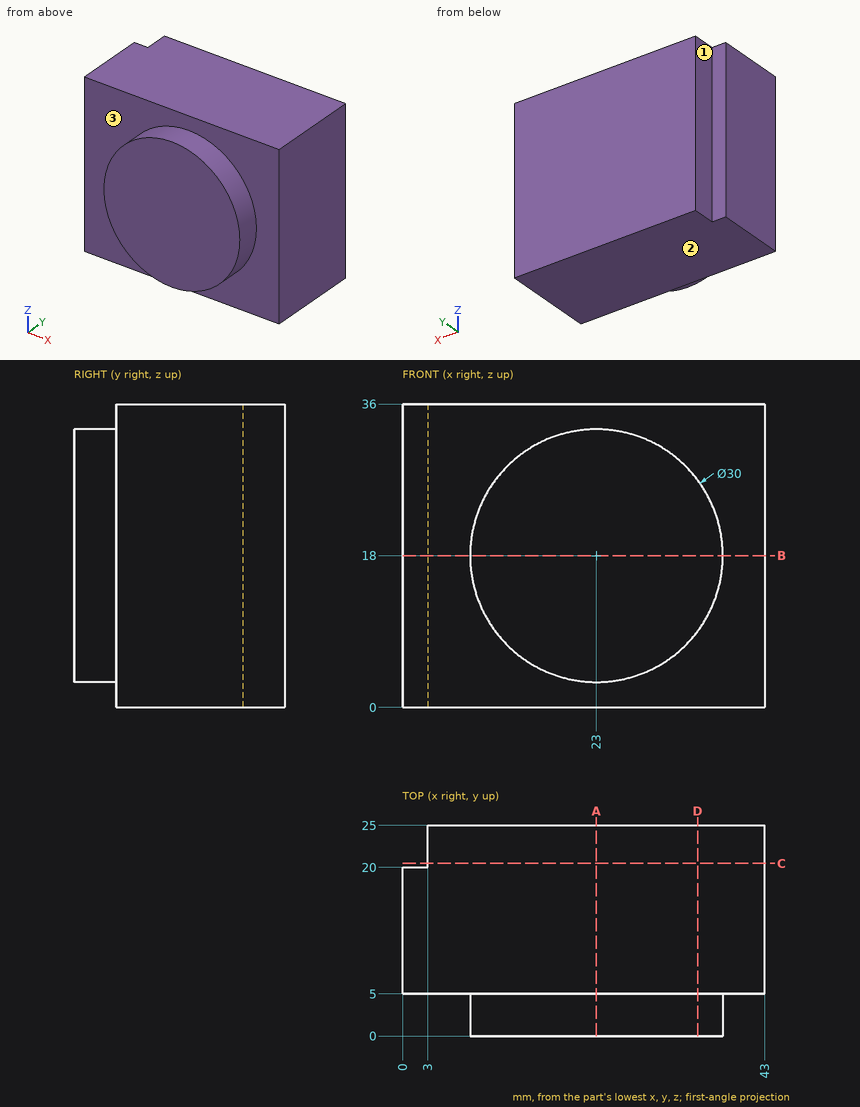
Can you work these out from the drawing? Everything is in mm from the part's minimum corner. A direction names the side the tool comes from. Coordinates: 2 decimals unless noted, no trailing zeros. Loops run counter-clockwise (first coordinate to the right, second up) from the corner with the lowest first, then second, coordinate; pieces in that order, holes last. Notation, with made-up numbers: (-22.75, 17.25) -> (-6.75, 17.25) arc R16 ccw to (-6.75, 40.25) -> close; hole circle Ø9 at (33.25, 71). An arc over 180 degrees is marked (long way). Return JSON: item names as keys, results as strings.
1) If we section it at B-B, the plane z = 18: Write out the boundary of the cut face in (x, y), then the cut area to 3 significant figures.
Results below:
{"outline": "(0, 5) -> (8, 5) -> (8, 0) -> (38, 0) -> (38, 5) -> (43, 5) -> (43, 25) -> (3, 25) -> (3, 20) -> (0, 20) -> close", "area": "995 mm²"}
2) Will these pins go through, and if not, where does the flat tip stop? pin 1 (3.5 mm diameter, centred on x = 1, z = 14, fed in from +Y); pin 2 (4 mm diameter, centred on y = 22.5, z = 11, fed in from -X).
Results below:
{"pin 1": "y = 20", "pin 2": "x = 3"}
3) If we section it at A-A, the plane x = 23: Write out the boundary of the cut face in (y, z).
Results below:
{"outline": "(0, 3) -> (5, 3) -> (5, 0) -> (25, 0) -> (25, 36) -> (5, 36) -> (5, 33) -> (0, 33) -> close"}
4) If we section it at D-D, the plane x = 35: Write out the boundary of the cut face in (y, z).
Results below:
{"outline": "(0, 9) -> (5, 9) -> (5, 0) -> (25, 0) -> (25, 36) -> (5, 36) -> (5, 27) -> (0, 27) -> close"}
5) I need wall thicknesses on line 1 (Y direction, x = 8, z = 28); line 2 (X direction, y = 3.75, z = 22.5); line 3 (Z direction, x = 21.5, y = 2). Which ranges of each line are inside material? Lowest first, please. Write a range as from..to.
Results below:
{"line 1": "5..25", "line 2": "8.69..37.31", "line 3": "3.08..32.92"}
6) For the marked faces 1, 2 and 3, which set-ups out of +Z, -Z, +X, -X, +Y, -Y let a thin tool reach every point of the face, with its end or its side?
Results below:
{"face 1": "+Z, -Z, -X, +Y", "face 2": "-Z, +X, -X, +Y, -Y", "face 3": "-Y"}
7) If we section it at C-C, the plane y = 20.5: Write out the boundary of the cut face in (x, z).
Results below:
{"outline": "(3, 0) -> (43, 0) -> (43, 36) -> (3, 36) -> close"}
